from build123d import *

# Parameters (mm, degrees)
F0_W      = 139.7
F0_H      = 38.1
F1_DEPTH  = 1828.8
F3_W      = 331.3202857971
F3_H      = 260.5838701129
F4_DEPTH  = 101.6
F7_W      = 1553.4552037716
F7_H      = 1155.3529500961
F8_DEPTH  = 762
F9_R      = 6.35
F10_DEPTH = 38.101


# Not quite as in the source:
# - a feature names something its author has since deleted; it is built from what else it names


with BuildPart() as f1:
    # F0 (on Front) → F1 (new body)
    with BuildSketch(Plane.XZ):
        with Locations((69.85, 19.05)):
            Rectangle(F0_W, F0_H)
    extrude(amount=F1_DEPTH)

    # F3 (on face) → F4 (cut)
    with BuildSketch(Plane(origin=(984.25, -984.25, 0), x_dir=(-0.7071067812, -0.7071067812, 0), z_dir=(-0.7071067812, 0.7071067812, 0))):
        with Locations((1222.6701974869, 7.0506222546)):
            Rectangle(F3_W, F3_H)
    extrude(amount=F4_DEPTH, mode=Mode.SUBTRACT)

    # F7 (on face) → F8 (cut)
    with BuildSketch(Plane(origin=(-315.2209189803, -315.2209189803, 0), x_dir=(0.7071067812, -0.7071067812, 0), z_dir=(-0.7071067812, -0.7071067812, 0))):
        with Locations((614.4417077303, -181.5140247345)):
            Rectangle(F7_W, F7_H)
    extrude(amount=-F8_DEPTH, mode=Mode.SUBTRACT)

    # F9 (on face) → F10 (cut, through all)
    with BuildSketch(Plane.XY.offset(38.1)):
        with Locations((69.85, -833.6418379607)):
            Circle(F9_R)
    extrude(amount=-F10_DEPTH, mode=Mode.SUBTRACT)


solid = f1.part
Geometry check sheet. Reference: the model listing, model coordinates, mm. Give positions to 0.01 mm unless a question says otherwise; leave off trailing zeros. Order: outer loops, then holes, each group sorted by start corner. A loop starts at its lowest first (then second) coordinate and runs counter-clockwise, first axis right, second up.
1) Cross-section at B-B (x = 36.5). Record the boundary of the cut face in (y, z), then the cut area to 3 significant figures.
Results are:
outline: (-1788.32, 0) - (-666.94, 0) - (-666.94, 38.1) - (-1788.32, 38.1) - close
area: 42,700 mm2
2) Cross-section at A-A (z = 17). Record the boundary of the cut face in (x, y).
Results are:
outline: (0, -1824.82) - (139.7, -1685.12) - (139.7, -770.14) - (0, -630.44) - close; hole circle Ø12.7 at (69.85, -833.64)
3) Material ranges on probe 1 along Y at (x, z) = (69, 11); probe 2 along Y at (x, z) = (69.85, 11); probe 3 along Y at (x, z) = (105, 14), recorded low to high.
Results are:
probe 1: y = -1755.82 to -839.93, -827.35 to -699.44
probe 2: y = -1754.97 to -839.99, -827.29 to -700.29
probe 3: y = -1719.82 to -735.44
4) Cross-section at C-C (y = -1714). Record the boundary of the cut face in (x, z), then the cut area to 3 significant figures.
Results are:
outline: (0, 0) - (110.82, 0) - (110.82, 38.1) - (0, 38.1) - close
area: 4,220 mm2
5) Gauge pin test, flat ends, axial feed: pin 1 (12 mm diameter, centred on x = 61, z = 33, fed in from +Y); pin 2 (10 mm diameter, centred on x = 60.5, z = 4, fed in from +Y); pin 3 (11.5 mm diameter, centred on x = 69.85, y = -833.64, fed in from -Z); pin 4 (2 mm diameter, centred on x = 66.5, z = 33.5, fed in from -Y). Record the tip position at first contact, or that the pin passes through.
Results are:
pin 1: stops at y = -685.44
pin 2: stops at y = -685.94
pin 3: passes through
pin 4: stops at y = -1759.32
